Read the model definition and answer for the solid it produces. Units are mm, in the model's axes. Face numbers are marked on the shaded views. A direction names the side the tool comes from. Give positions to 0.01 mm unless a question says otherwise; leave off trailing zeros. Write each loop counter-clockwise with the first axis right and the second up, starting at its lowest first coordinate (ties: lowest second). Pieces come first, ordered by that corner, then holes. Notation, with made-up numbers: (-32, 11) -> (22, 11) arc R20 ccw to (22, 26) -> close; hole circle Ø5 at (20, 31). An arc over 180 degrees is marked (long way). Use a Markdown table: item, result.
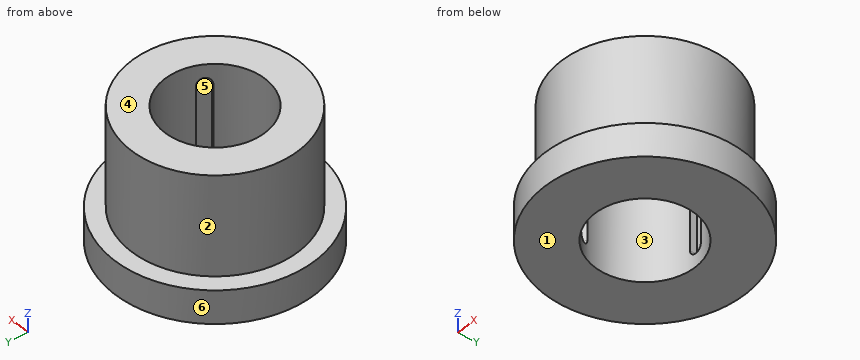
Autodesk Inventor part; units mm, degrees
ref_plane "Work Plane1" through (0, 8.5, 0) normal (0, 1, 0) x (-1, 0, 0)
ref_plane "YZ Plane" through (0, 0, 0) normal (1, 0, 0) x (0, 1, 0)
ref_plane "XY Plane" through (0, 0, 0) normal (0, 0, 1) x (1, 0, 0)
sketch "Sketch1" plane through (0, 0, 0) normal (0, 1, 0) x (-1, 0, 0)
  line L0 (0, 0) -> (15, 0)
  line L1 (15, 0) -> (15, 20)
  line L2 (15, 20) -> (0, 20)
  line L3 (0, 20) -> (0, 0)
  line L4 (12.5, 20) -> (12.5, 5)
  line L5 (12.5, 5) -> (15, 5)
  line L6 (7.5, 20) -> (7.5, 0)
  dimension "d1" = 30
  dimension "d2" = 25
  dimension "d3" = 15
  dimension "d4" = 5
  dimension "d5" = 15
revolve "Revolution1" add sketch "Sketch1" angle 360 about axis through (0, 0, 20) along (0, 0, -1) contours L6 L2 L4 L5 L1 L0
ref_plane "Work Plane1" through (0, 8.5, 0) normal (0, 1, 0) x (-1, 0, 0)
sketch "Sketch2" plane through (0, 8.5, 0) normal (0, 1, 0) x (-1, 0, 0)
  line L0 (0, 18) -> (0, 2) construction
  line L1 (1, 17) -> (1, 3)
  line L2 (-1, 3) -> (-1, 17)
  arc A0 (1, 17) -> (-1, 17) centre (0, 17) ccw
  arc A1 (-1, 3) -> (1, 3) centre (0, 3) ccw
  line L3 (-12.5, 20) -> (12.5, 20) construction
  point P0 (0, 0)
  point P1 (0, 10)
  point P2 (0, 18)
  dimension "d8" = 16
  dimension "d9" = 2
  dimension "d10" = 2
extrude "Extrusion1" cut sketch "Sketch2" against normal up to surface
pattern_circular "Circular Pattern1" count 3 over 360 about axis through (0, 0, -10) along (0, 0, 1) of "Extrusion1"
properties material "Bronze, Soft Tin"
Item 1: Each of these flat-tipped pins is pushed along its axis until it touches: P1, Ø10, axis at x = -1.5, y = 0.5, coming from the +Z side; P2, Ø1.5, axis at x = -0.5, z = 14, coming from the +Y side; P3, Ø1.2, axis at y = 8, z = 13, coming from the -X side; P4, Ø2, axis at x = 0, z = 7.5, coming from the -Y side. Where does it stop, or does it pass through?
Return value:
| item | result |
|---|---|
| P1 | through |
| P2 | y = 12.5 |
| P3 | x = -10.07 |
| P4 | y = -12.5 |
Item 2: A cutting plane is placed at B-B (z = 14.5). Give the vertices of the cut face in (x, y), then the cut area to 3 significant figures.
Return value:
| item | result |
|---|---|
| outline | circle Ø25 at (0, 0); hole (-7.86, -3.38) -> (-6.86, -5.12) -> (-5.94, -4.58) arc R7.5 ccw to (5.94, -4.58) -> (6.86, -5.12) -> (7.86, -3.38) -> (6.94, -2.85) arc R7.5 ccw to (1, 7.43) -> (1, 8.5) -> (-1, 8.5) -> (-1, 7.43) arc R7.5 ccw to (-6.94, -2.85) -> close |
| area | 308 mm^2 |
Item 3: Straight lines are drawn through the part: line 1 along Y through (x, z) = (0, 14); line 2 along Z through (x, y) = (-7.5, 12); line 3 along Y through (x, z) = (-10, 8). For each, find the intervals that lie inside material, in ascending order. Write a range as [from, to].
Return value:
| item | result |
|---|---|
| line 1 | [-12.5, -7.5], [8.5, 12.5] |
| line 2 | [0, 5] |
| line 3 | [-7.5, 7.5] |
Item 4: For a pull along Y with two mould halves and no side action, classify the marked faces 3, 4, 5 and 6 as +Y half, -Y half, draft (parallel to the pull), parting line (faces both ways), or undercut.
Return value:
| item | result |
|---|---|
| face 3 | undercut |
| face 4 | draft |
| face 5 | undercut |
| face 6 | parting line |
Item 5: A cutting plane is placed at D-D (y = 10.75). Give the vertices of the cut face in (x, z).
Return value:
| item | result |
|---|---|
| outline | (-10.46, 0) -> (10.46, 0) -> (10.46, 5) -> (6.38, 5) -> (6.38, 20) -> (-6.38, 20) -> (-6.38, 5) -> (-10.46, 5) -> close |
Item 6: A cutting plane is placed at A-A (y = 0). Give the vertices of the cut face in (x, z), then the cut area to 3 significant figures.
Return value:
| item | result |
|---|---|
| outline | (-15, 0) -> (-7.5, 0) -> (-7.5, 20) -> (-12.5, 20) -> (-12.5, 5) -> (-15, 5) -> close; (7.5, 0) -> (15, 0) -> (15, 5) -> (12.5, 5) -> (12.5, 20) -> (7.5, 20) -> close |
| area | 225 mm^2 |
Item 7: A tool of negligible diameter and unlimited length cuts with its end or side. For the marked faces 1 and 2, from which of +Z, -Z, +X, -X, +Y, -Y can it reach the whole face along a straight path? Write none if from no direction.
Return value:
| item | result |
|---|---|
| face 1 | -Z, +X, -X, +Y, -Y |
| face 2 | +Z |
Item 8: A cutting plane is placed at C-C (x = -1.5). Give the vertices of the cut face in (y, z).
Return value:
| item | result |
|---|---|
| outline | (-14.92, 0) -> (-7.35, 0) -> (-7.35, 20) -> (-12.41, 20) -> (-12.41, 5) -> (-14.92, 5) -> close; (7.35, 0) -> (14.92, 0) -> (14.92, 5) -> (12.41, 5) -> (12.41, 20) -> (7.35, 20) -> close |
